Design review of the part built by this model. Coordinates are the model's own, in mm. Face numbers are marked on the shaded views. A direction names the side the tool comes from. Coordinates: 2 decimals unless noted, no trailing zeros. Loops run counter-clockwise (first coordinate to the right, second up) from the corner with the lowest first, then second, coordinate; pieces in that order, holes last. Notation, with made-up numbers: (-33.5, 18) - (20.5, 18) arc R35 cw to (20.5, 51) - close; hole circle Ø1 at (-8.5, 74). An arc over 180 degrees is marked (long way). Use one line per item in the form item = value. Start each with the question number.
(1) For L1, parallel to X at y = 4, z = 9; L2, parallel to Y at x = -188.5, z = 3.5; L3, parallel to Z at x = 102, y = -13.5, list the stretches that pass through material, from the lowest coordinate up.
(2) Clearance check with flat-ended pins moving along their axes: pin 1 Ø2 at (x, z) = (-136, 0.5) entering from -Y; pin 2 Ø9.5 at (x, y) = (17.5, 5.5) entering from +Z; pin 3 Ø6 at (x, z) = (-88.5, 39.5) entering from +Y. State where each tip first meets the part, or that it passes through.
(3) Add section A-A (y = 2). State the section outline as (x, z) points, plus the area to 3 significant figures.
(4) Tool access review of the marked faces 4 and 5: name each direction out of +Z, -Z, +X, -X, +Y, -Y from which nothing blocks a thin tool from reaching the whole face with its end or side.
(5) The part is to be moulded in two halves that separate along Y. For the marked faces 1, 2 and 3, say which applies: pulls with the +Y half, pulls with the -Y half, needs draft (parallel to the pull), parting line crosses it, or undercut.
(6) Add section C-C (z = 37). State the section outline as (x, y) points.
(7) Add section D-D (x = -125). State the section outline as (y, z) points.
(8) Add section B-B (x = 115). State the section outline as (y, z) points, plus the area to 3 significant figures.
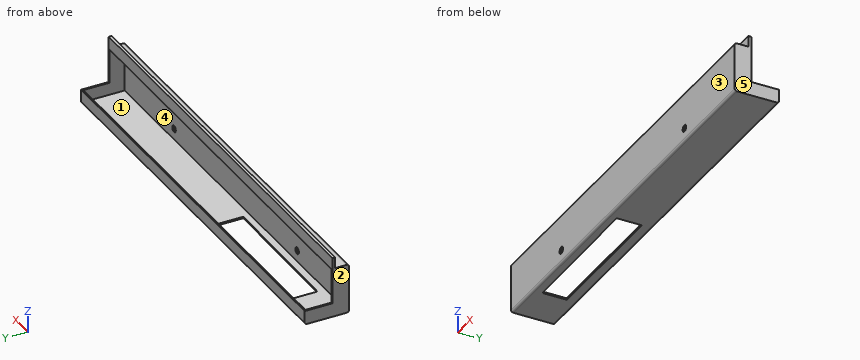
```python
from build123d import *

# Parameters (mm, degrees)
SKETCH1_W           = 482.6
SKETCH1_H           = 50.8
BOSS_EXTRUDE1_DEPTH = 69.85
CUT_EXTRUDE2_DEPTH  = 49.022
SKETCH3_W           = 482.6
SKETCH3_H           = 16.002
CUT_EXTRUDE3_DEPTH  = 31.75
SKETCH4_W           = 482.6
SKETCH4_H           = 15.748
CUT_EXTRUDE4_DEPTH  = 12.7
SHELL2_START        = -23.622
SHELL2_OUTLINE_W    = 479.044
SHELL2_OUTLINE_H    = 14.224
SHELL2_DEPTH        = 47.244
SKETCH5_W           = 1.778
SKETCH5_H           = 17.272
BOSS_EXTRUDE2_DEPTH = 44.45
FILLET1_R           = 2.54
SKETCH6_R           = 3.81
CUT_EXTRUDE5_DEPTH  = 44.45
CUT_EXTRUDE6_REACH  = 254.487


# Read off the part's stored shape, not the designer's step: Shell2
with BuildPart() as part:
    # Sketch1 → Boss-Extrude1 (new body)
    with BuildSketch(Plane.XY):
        Rectangle(SKETCH1_W, SKETCH1_H)
    extrude(amount=BOSS_EXTRUDE1_DEPTH)

    # Sketch2 → Cut-Extrude2 (cut)
    with BuildSketch(Plane(origin=(0, 25.4, 0), x_dir=(1, 0, 0), z_dir=(0, 1, 0))):
        Polygon((241.3, -16.002), (-241.3, -16.002), (-241.3, -34.925), (-241.3, -53.848), (241.3, -53.848), align=None)
    extrude(amount=-CUT_EXTRUDE2_DEPTH, mode=Mode.SUBTRACT)

    # Sketch3 → Cut-Extrude3 (cut)
    with BuildSketch(Plane(origin=(0, 25.4, 0), x_dir=(1, 0, 0), z_dir=(0, 1, 0))):
        with Locations((0, -61.849)):
            Rectangle(SKETCH3_W, SKETCH3_H)
    extrude(amount=-CUT_EXTRUDE3_DEPTH, mode=Mode.SUBTRACT)

    # Sketch4 → Cut-Extrude4 (cut)
    with BuildSketch(Plane.XY.offset(69.85)):
        with Locations((0, -17.526)):
            Rectangle(SKETCH4_W, SKETCH4_H)
    extrude(amount=-CUT_EXTRUDE4_DEPTH, mode=Mode.SUBTRACT)

    # Shell2 outline → Shell2 (cut)
    with BuildSketch(Plane(origin=(0, 0, 0), x_dir=(1, 0, 0), z_dir=(0, 1, 0)).offset(SHELL2_START)):
        with Locations((0, -8.89)):
            Rectangle(SHELL2_OUTLINE_W, SHELL2_OUTLINE_H)
    extrude(amount=SHELL2_DEPTH, mode=Mode.SUBTRACT)

    # Sketch5 → Boss-Extrude2 (add)
    with BuildSketch(Plane(origin=(0, 0, 53.848), x_dir=(-1, 0, 0), z_dir=(0, 0, -1))):
        with Locations((240.411, -14.986)):
            Rectangle(SKETCH5_W, SKETCH5_H)
        with Locations((-240.411, -14.986)):
            Rectangle(SKETCH5_W, SKETCH5_H)
    extrude(amount=BOSS_EXTRUDE2_DEPTH)

    # Fillet1
    fillet1_edges = [part.edges().sort_by_distance(p)[0] for p in [
        (0, -25.4, 0),
        (0, -25.4, 57.15),
        (0, 25.4, 0),
        (0, -6.35, 53.848),
    ]]
    fillet(fillet1_edges, radius=FILLET1_R)

    # Sketch6 → Cut-Extrude5 (cut)
    with BuildSketch(Plane(origin=(0, -23.622, 0), x_dir=(1, 0, 0), z_dir=(0, 1, 0))):
        with Locations(Location((-132.842, -14.478, 0), (0, 0, 270))):
            Circle(SKETCH6_R)
        with Locations(Location((132.842, -14.478, 0), (0, 0, 270))):
            Circle(SKETCH6_R)
    extrude(amount=-CUT_EXTRUDE5_DEPTH, mode=Mode.SUBTRACT)

    # Sketch8 → Cut-Extrude6 (cut, up to next)
    with BuildSketch(Plane(origin=(0, 0, 0), x_dir=(-1, 0, 0), z_dir=(0, 0, -1)), mode=Mode.PRIVATE) as cut_extrude6_sk1:
        Polygon((31.482, 13.4), (31.482, -15.81), (193.836883288, -14.551149116), (193.836883288, 13.4), align=None)
    cut_extrude6_tool1 = extrude(cut_extrude6_sk1.sketch, amount=-CUT_EXTRUDE6_REACH, mode=Mode.PRIVATE) & part.part
    add(cut_extrude6_tool1.solids().sort_by_distance((-112.063522, -0.892598, 0))[0], mode=Mode.SUBTRACT)


solid = part.part
```
Computed values:
q1.L1 = -241.3 to -239.52, 239.52 to 241.3
q1.L2 = -25.4 to -23.62, 23.62 to 25.4
q1.L3 = 0 to 1.78, 53.85 to 57.15
q2.pin_1 = -25.18
q2.pin_2 = 1.78
q2.pin_3 = -23.62
q3.outline = (-241.3, 0) - (-193.84, 0) - (-193.84, 1.78) - (-239.52, 1.78) - (-239.52, 16) - (-241.3, 16) - close; (-31.48, 0) - (241.3, 0) - (241.3, 16) - (239.52, 16) - (239.52, 1.78) - (-31.48, 1.78) - close
q3.area = 620 mm^2
q4.face_4 = none
q4.face_5 = +Z, -Z, +X, +Y, -Y
q5.face_1 = undercut
q5.face_2 = needs draft
q5.face_3 = pulls with the -Y half
q6.outline = (-241.3, -25.4) - (241.3, -25.4) - (241.3, -6.35) - (239.52, -6.35) - (239.52, -23.62) - (-239.52, -23.62) - (-239.52, -6.35) - (-241.3, -6.35) - close
q7.outline = (-25.4, 2.54) arc R2.54 ccw to (-22.86, 0) - (-15.08, 0) - (-15.08, 1.78) - (-23.62, 1.78) - (-23.62, 53.85) - (-8.89, 53.85) arc R2.54 ccw to (-6.35, 56.39) - (-6.35, 69.85) - (-9.65, 69.85) - (-9.65, 57.15) - (-22.86, 57.15) arc R2.54 ccw to (-25.4, 54.61) - close; (13.4, 0) - (22.86, 0) arc R2.54 ccw to (25.4, 2.54) - (25.4, 16) - (23.62, 16) - (23.62, 1.78) - (13.4, 1.78) - close
q8.outline = (-25.4, 2.54) arc R2.54 ccw to (-22.86, 0) - (22.86, 0) arc R2.54 ccw to (25.4, 2.54) - (25.4, 16) - (23.62, 16) - (23.62, 1.78) - (-23.62, 1.78) - (-23.62, 53.85) - (-8.89, 53.85) arc R2.54 ccw to (-6.35, 56.39) - (-6.35, 69.85) - (-9.65, 69.85) - (-9.65, 57.15) - (-22.86, 57.15) arc R2.54 ccw to (-25.4, 54.61) - close
q8.area = 307 mm^2
